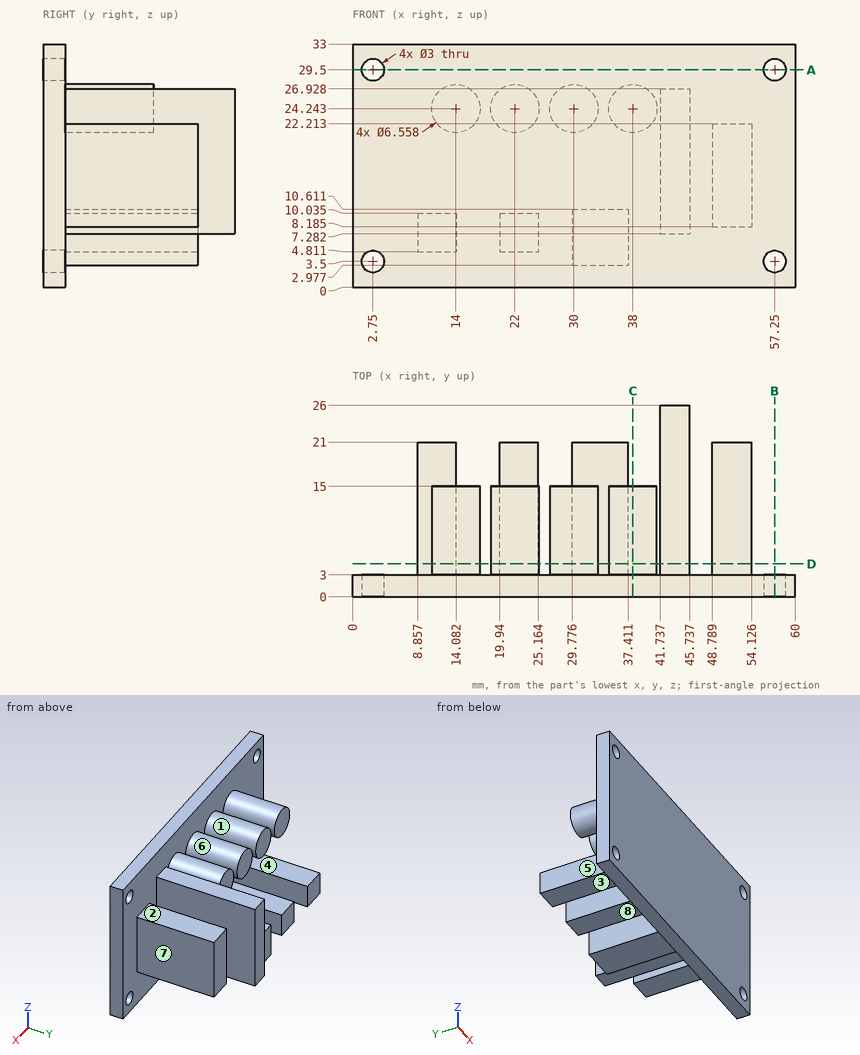
For this review, use the dimensioned drawing (mm, ordinates from the lowest corner) and the shaded views. A direction names the side the tool comes from. Round coordinates to 2 decimals unless told otherwise and drop trailing zeros. Write each loop counter-clockwise with the first axis right and the second up, starting at its lowest first coordinate (ties: lowest second). Pieces come first, ordered by that corner, then holes. Notation, with made-up numbers: (49.5, 29) -> (65.5, 29) arc R19 cw to (65.5, 47) -> close; hole circle Ø3 at (-21.75, 71.5). An arc over 180 degrees is marked (long way). Use CSV: the item, a comma, the result in double quotes.
(1) Clearance check with flat-ended pins moving along their axes: P1, Ø2.5, axis at y = 16, z = 7, coming from the -X side; P2, Ø5, axis at x = 34, z = 18.5, coming from the -Y side; P3, Ø8.5, axis at y = 9, z = 6, coming from the +X side; P4, Ø2, axis at x = 13.5, z = 25.5, coming from the +Y side. State where each tip first meets the part, or that it passes through.
Computed values:
P1,"x = 8.86"
P2,"y = 0"
P3,"x = 54.13"
P4,"y = 15"
(2) To check wall thickness, follow L1, parallel to Z at x = 2.75, y = 0.7; L2, parallel to X at y = 1.75, z = 3.5; L3, parallel to X at y = 18.75, z = 18. State the ranges of each line that lie inside material, in increasing order. Write a range as [from, to].
Computed values:
L1,"[0, 2], [5, 28], [31, 33]"
L2,"[0, 1.25], [4.25, 55.75], [58.75, 60]"
L3,"[41.74, 45.74], [48.79, 54.13]"
(3) For the marked faces 1, 2, 3, 4 and 5, list the 3-axis set-ups (+Z, -Z, +X, -X, +Y, -Y) from which the entire face can be reached by the end or side of a thin tool; tool diameter is ignored.
Computed values:
face 1,"+Y"
face 2,"+Z, +X, +Y"
face 3,"-Z, -X, +Y"
face 4,"-X, +Y"
face 5,"+Z, -Z, -X, +Y"
(4) Draft analysis for pull direction Z (two halves, no side actions). For the marked faces 6, 7 and 8, state which applies: +Z half, -Z half, draft (parallel to the pull), parting line (faces both ways), or undercut.
Computed values:
face 6,"undercut"
face 7,"draft"
face 8,"-Z half"
(5) Consider section B-B, the plane x = 57.25. Give the boundary of the cut face in (y, z).
Computed values:
outline,"(0, 0) -> (3, 0) -> (3, 2) -> (0, 2) -> close; (0, 5) -> (3, 5) -> (3, 28) -> (0, 28) -> close; (0, 31) -> (3, 31) -> (3, 33) -> (0, 33) -> close"
(6) Consider section C-C, the plane x = 38. Give the boundary of the cut face in (y, z) (1 decimal).
Computed values:
outline,"(0, 0) -> (3, 0) -> (3, 21) -> (15, 21) -> (15, 27.5) -> (3, 27.5) -> (3, 33) -> (0, 33) -> close"
(7) Consider section D-D, the plane y = 4.5. Give the number of separate pieces and of enclosed holes in the cut face.
Computed values:
separate pieces,"9"
enclosed holes,"0"
(8) Consider section A-A, the plane z = 29.5. Give the boundary of the cut face in (x, y).
Computed values:
outline,"(0, 0) -> (1.25, 0) -> (1.25, 3) -> (0, 3) -> close; (4.25, 0) -> (55.75, 0) -> (55.75, 3) -> (4.25, 3) -> close; (58.75, 0) -> (60, 0) -> (60, 3) -> (58.75, 3) -> close"
